from build123d import *

# Parameters (mm, degrees)
SKICA1_W                = 95
SKICA1_H                = 50
P_IDAT_VYSUNUT_M1_DEPTH = 1.2
SKICA2_W                = 95
SKICA2_H                = 50
SKICA2_W_2              = 92.6
SKICA2_H_2              = 47.6
P_IDAT_VYSUNUT_M2_DEPTH = 4
P_IDAT_VYSUNUT_M3_DEPTH = 8


with BuildPart() as part:
    # Skica1 → Přidat vysunutím1 (new body)
    with BuildSketch(Plane.XY):
        with Locations((47.5, 25)):
            Rectangle(SKICA1_W, SKICA1_H)
    extrude(amount=P_IDAT_VYSUNUT_M1_DEPTH)

    # Skica2 → Přidat vysunutím2 (add)
    with BuildSketch(Plane.XY.offset(1.2)):
        with Locations((47.5, 25)):
            Rectangle(SKICA2_W, SKICA2_H)
        with Locations((47.5, 25)):
            Rectangle(SKICA2_W_2, SKICA2_H_2, mode=Mode.SUBTRACT)
    extrude(amount=P_IDAT_VYSUNUT_M2_DEPTH)

    # Skica3 → Přidat vysunutím3 (add)
    with BuildSketch(Plane.XY.offset(1.2)):
        Polygon((1.2, 48.8), (6.2, 48.8), (1.2, 43.8), align=None)
        Polygon((93.8, 48.8), (93.8, 43.8), (88.8, 48.8), align=None)
        Polygon((93.8, 1.2), (88.8, 1.2), (93.8, 6.2), align=None)
        Polygon((1.2, 1.2), (1.2, 6.2), (6.2, 1.2), align=None)
    extrude(amount=P_IDAT_VYSUNUT_M3_DEPTH)


solid = part.part
Input: part model. Units: mm. Frame: model coordinates. A direction names the side the tool comes from. Round coordinates to 2 decimals unless told otherwise and drop trailing zeros. Order: outer loops, then holes, each group sorted by start corner. A loop starts at its lowest first (then second) coordinate and runs counter-clockwise, first axis right, second up. Notation, with made-up numbers: (81.5, 89.25) - (140.5, 89.25) arc R18 ccw to (140.5, 109.25) - close; hole circle Ø10 at (-4, 77.5). An arc over 180 degrees is marked (long way). Answer as a JSON object with one key per item and string values. Group by question number.
(1) Cut plane C-C (x = 42). Return loops of the section in (y, z), then the cut area to 3 significant figures.
(2) Cut plane B-B (y = 8). Return loops of the section in (x, z), then the cut area to 3 significant figures.
(3) Cut plane D-D (y = 46). Return loops of the section in (x, z), then the cut area to 3 significant figures.
(4) Material intervals for probe 1 along Y at (x, z) = (53, 2); probe 2 along X at (y, z) = (21, 3.25); probe 3 along Z at (x, y) = (8.5, 7), sorted ascending. Write a range as from..to.
(5) Reachability of faces 4 (the face through (1.2, 46, 7)), 5 (the face through (93.8, 4, 7)), 6 (the face through (47, 1.2, 3)), 7 (the face through (91, 48.8, 7)), 8 (the face through (91, 1.2, 7)) from +Z, -Z, +X, -X, +Y, -Y: full face, straight path, thin tool, end or side. Return the list, or none.
(6) Draft query along X for faces 1 (the face through (92, 47, 9.2)), 2 (the face through (0, 25, 3)), 3 (the face through (3.7, 3.7, 5.1)). Return one class per face: released by +X, released by -X, zero draft, split by the parting line, or undercut.
(7) Pin query (flat end, axial travel): P1, Ø4.5, axis at y = 3.5, z = 8, coming from the +X side; P2, Ø2, axis at y = 3.5, z = 6.5, coming from the -X side; P3, Ø4.5, axis at x = 90.5, z = 8, coming from the -Y side. Return the tip coordinate at first contact, or that it passes through.
(8) Cut plane A-A (z = 6.75). Return loops of the section in (x, y).
Here are the results:
{
 "1": {"outline": "(0, 0) - (50, 0) - (50, 5.2) - (48.8, 5.2) - (48.8, 1.2) - (1.2, 1.2) - (1.2, 5.2) - (0, 5.2) - close", "area": "69.6 mm^2"},
 "2": {"outline": "(0, 0) - (95, 0) - (95, 5.2) - (93.8, 5.2) - (93.8, 1.2) - (1.2, 1.2) - (1.2, 5.2) - (0, 5.2) - close", "area": "124 mm^2"},
 "3": {"outline": "(0, 0) - (95, 0) - (95, 5.2) - (93.8, 5.2) - (93.8, 9.2) - (91.6, 9.2) - (91.6, 1.2) - (3.4, 1.2) - (3.4, 9.2) - (1.2, 9.2) - (1.2, 5.2) - (0, 5.2) - close", "area": "159 mm^2"},
 "4": {"probe 1": "y = 0..1.2, 48.8..50", "probe 2": "x = 0..1.2, 93.8..95", "probe 3": "z = 0..1.2"},
 "5": {"face 4": "+Z, -X, +Y, -Y", "face 5": "+Z, +X, +Y, -Y", "face 6": "+Z", "face 7": "+Z, +X, -X, +Y", "face 8": "+Z, +X, -X, -Y"},
 "6": {"face 1": "zero draft", "face 2": "released by -X", "face 3": "undercut"},
 "7": {"P1": "stops at x = 93.8", "P2": "stops at x = 1.2", "P3": "stops at y = 1.2"},
 "8": {"outline": "(1.2, 1.2) - (6.2, 1.2) - (1.2, 6.2) - close; (1.2, 43.8) - (6.2, 48.8) - (1.2, 48.8) - close; (88.8, 1.2) - (93.8, 1.2) - (93.8, 6.2) - close; (88.8, 48.8) - (93.8, 43.8) - (93.8, 48.8) - close"}
}
